Could you check a few things on this model? Use its own coordinates, in mm. A direction names the side the tool comes from. Coordinates: 2 decimals unless noted, no trailing zeros. Order: outer loops, then holes, each group sorted by start corner. A loop starts at its lowest first (then second) coordinate and runs counter-clockwise, first axis right, second up.
```python
from build123d import *

# Parameters (mm, degrees)
SKETCH2_W          = 3.5
SKETCH2_H          = 2.5
CUT_EXTRUDE1_DEPTH = 3.5
FILLET1_R          = 1.25
CUT_EXTRUDE2_DEPTH = 14.37908816


with BuildPart() as part:
    # Sketch1 → Revolve1 (revolve)
    with BuildSketch(Plane.XY, mode=Mode.PRIVATE) as revolve1_sk:
        Polygon((0, 9), (4, 9), (4, 3), (7, 3), (7, 0), (0, 0), align=None)
    revolve(revolve1_sk.sketch.rotate(Axis((0, 9, 0), (0, -1, 0)), 180), axis=Axis((0, 9, 0), (0, -1, 0)))

    # Sketch2 → Cut-Extrude1 (cut)
    with BuildSketch(Plane.XZ):
        Rectangle(SKETCH2_W, SKETCH2_H)
    extrude(amount=-CUT_EXTRUDE1_DEPTH, mode=Mode.SUBTRACT)

    # Fillet1
    fillet1_edges = [part.edges().sort_by_distance(p)[0] for p in [
        (4, 9, 0),
    ]]
    fillet(fillet1_edges, radius=FILLET1_R)

    # Sketch3 → Cut-Extrude2 (cut, through all)
    with BuildSketch(Plane(origin=(0, 0, 0), x_dir=(1, 0, 0), z_dir=(0, 1, 0))):
        with BuildLine():
            Line((-14, -3), (-14, 3))
            ThreePointArc((-14, 3), (0, 17), (14, 3))
            Line((14, 3), (14, -3))
            ThreePointArc((14, -3), (0, -17), (-14, -3))
        make_face()
        with BuildLine():
            Line((-4, -3), (-4, 3))
            ThreePointArc((-4, 3), (0, 7), (4, 3))
            Line((4, 3), (4, -3))
            ThreePointArc((4, -3), (0, -7), (-4, -3))
        make_face(mode=Mode.SUBTRACT)
    extrude(amount=CUT_EXTRUDE2_DEPTH, mode=Mode.SUBTRACT)


solid = part.part
```
Item 1: Suppose I cut it at B-B (x = 0). List the corners of the cut face in (y, z) for me.
Item 2: I need wall thicknesses on line 1 (Y direction, x = -1.5, z = 5.75); line 2 (Z direction, x = 0, y = 7.5); line 3 (Z direction, x = 1.5, y = 1.25). Which ranges of each line are inside material? Lowest first, please.
Item 3: Suppose I cut it at D-D (y = 8.25). List the corners of the cut face in (x, z) for me.
Item 4: Which directions (+Z, -Z, +X, -X, +Y, -Y) give clear straight access to the entire face, cutting with the end or side of a thin tool? Please do faces 1 (the face through (0.867, 5.342, 3.905)), 2 (the face through (1.75, 2, 0)), 3 (the face through (-4, 1, 0)).
Item 5: Suppose I cut it at A-A (y = 2.5). List the corners of the cut face in (x, z) for me.
Item 6: Suppose I cut it at C-C (y = 5.5). List the corners of the cut face in (x, z) for me, and give its area (3 significant figures).
Item 7: For pin 1 Ø4 at (y, z) = (5.5, 2) entering from -X; pin 2 Ø2 at (x, z) = (0, 0) entering from -Y; pin 3 Ø4 at (x, y) = (-0.5, 6.5) entering from -Z, each with a flat end and sliding along its axis, tell me the tip position at first contact or that it passes through.
Geometry results:
1. outline: (0, -7) - (3, -7) - (3, -4) - (7.75, -4) arc R1.25 ccw to (9, -2.75) - (9, 2.75) arc R1.25 ccw to (7.75, 4) - (3, 4) - (3, 7) - (0, 7) - (0, 1.25) - (3.5, 1.25) - (3.5, -1.25) - (0, -1.25) - close
2. line 1: y = 0 to 3
2. line 2: z = -4 to 4
2. line 3: z = -6.71 to -1.25, 1.25 to 6.71
3. outline: circle Ø7.79 at (0, 0)
4. face 1: +Y
4. face 2: -Y
4. face 3: +Z, -Z, -X, +Y, -Y
5. outline: (-4, -3) arc R4 ccw to (4, -3) - (4, 3) arc R4 ccw to (-4, 3) - close; hole (-1.75, -1.25) - (1.75, -1.25) - (1.75, 1.25) - (-1.75, 1.25) - close
6. outline: circle Ø8 at (0, 0)
6. area: 50.3 mm2
7. pin 1: stops at x = -4
7. pin 2: stops at y = 3.5
7. pin 3: stops at z = -4
